Source: CAD feature listing. Evaluate the final solid. Frame: model axes, mm. Face numbers are marked on the shaded views. A direction names the side the tool comes from. Give positions to 0.01 mm unless a question says otherwise; leave off trailing zeros. Loops run counter-clockwise (first coordinate to the right, second up) from the corner with the lowest first, then second, coordinate; pieces in that order, holes last. Notation, with made-up numbers: M 82,39.5 L 88,39.5 A4 cw 88,45.5 Z; hole C 69,18.5 d6. An arc over 180 degrees is marked long. Answer in a Markdown table with one row per item.
```python
from build123d import *

# Parameters (mm, degrees)
F0_R      = 9.525
F1_DEPTH  = 1.905
F2_DEPTH  = 11.43
F6_R      = 0.635
F7_DEPTH  = 2.54
F10_W     = 10.16
F10_H     = 1.27
F11_DEPTH = 3.81
F12_W     = 10.16
F12_H     = 1.905
F13_DEPTH = 3.81
F15_DEPTH = 0.254
F17_DEPTH = 0.254


with BuildPart() as f1:
    # F0 (on Top) → F1 (new body)
    with BuildSketch(Plane.XY):
        Polygon((12.573, 7.2590249345), (0, 14.518049869), (-12.573, 7.2590249345), (-12.573, -7.2590249345), (0, -14.518049869), (12.573, -7.2590249345), align=None)
        Circle(F0_R, mode=Mode.SUBTRACT)
        Circle(F0_R)
        with BuildLine():
            ThreePointArc((-6.985, -3.4925), (-9.2723234913, 0), (-6.985, 3.4925))
            Line((-6.985, 3.4925), (-6.985, -3.4925))
        make_face(mode=Mode.SUBTRACT)
        with BuildLine():
            Line((6.985, -3.4925), (6.985, 3.4925))
            ThreePointArc((6.985, 3.4925), (9.2723234913, 0), (6.985, -3.4925))
        make_face(mode=Mode.SUBTRACT)
    extrude(amount=F1_DEPTH)

    # F0 (on Top) → F2 (join)
    with BuildSketch(Plane.XY):
        with BuildLine():
            Line((-6.985, -3.4925), (-6.985, 3.4925))
            ThreePointArc((-6.985, 3.4925), (-9.2723234913, 0), (-6.985, -3.4925))
        make_face()
        with BuildLine():
            ThreePointArc((6.985, -3.4925), (9.2723234913, 0), (6.985, 3.4925))
            Line((6.985, 3.4925), (6.985, -3.4925))
        make_face()
    extrude(amount=F2_DEPTH)

    # F4 (on offset) → F5 (revolve)
    with BuildSketch(Plane.XY.offset(9.525)):
        with BuildLine():
            ThreePointArc((0, 7.112), (-7.112, 0), (0, -7.112))
            Line((0, -7.112), (0, 7.112))
        make_face()
    revolve(axis=Axis((0, 0, 9.525), (0, 1, 0)))

    # F6
    f6_edges = [f1.edges().sort_by_distance(p)[0] for p in [
        (-6.985, 0, 11.43),
        (-9.272323, 0, 11.43),
        (6.985, 0, 11.43),
        (9.272323, 0, 11.43),
    ]]
    fillet(f6_edges, radius=F6_R)

    # F0 (on Top) → F7 (join)
    with BuildSketch(Plane.XY):
        Circle(F0_R)
        with BuildLine():
            ThreePointArc((-6.985, -3.4925), (-9.2723234913, 0), (-6.985, 3.4925))
            Line((-6.985, 3.4925), (-6.985, -3.4925))
        make_face(mode=Mode.SUBTRACT)
        with BuildLine():
            Line((6.985, -3.4925), (6.985, 3.4925))
            ThreePointArc((6.985, 3.4925), (9.2723234913, 0), (6.985, -3.4925))
        make_face(mode=Mode.SUBTRACT)
    extrude(amount=F7_DEPTH)

    # F10 (on line) → F11 (cut, symmetric)
    with BuildSketch(Plane(origin=(0, -2.38125, 8.8869459855), x_dir=(1, 0, 0), z_dir=(0, -0.2588190451, 0.9659258263))):
        with Locations((0, -4.318)):
            Rectangle(F10_W, F10_H)
    extrude(amount=F11_DEPTH, both=True, mode=Mode.SUBTRACT)

    # F12 (on line) → F13 (cut, symmetric)
    with BuildSketch(Plane(origin=(0, 2.38125, 8.8869459855), x_dir=(1, 0, 0), z_dir=(0, -0.2588190451, -0.9659258263))):
        with Locations((0, 9.4615)):
            Rectangle(F12_W, F12_H)
    extrude(amount=F13_DEPTH, both=True, mode=Mode.SUBTRACT)

    # F14 (on face) → F15 (cut)
    with BuildSketch(Plane(origin=(0, -3.5575048182, -0.9532305431), x_dir=(1, 0, 0), z_dir=(0, -0.9659258263, -0.2588190451))):
        with BuildLine():
            Line((3.0137271476, 10.2578568757), (-3.0137271476, 10.2578568757))
            ThreePointArc((-3.0137271476, 10.2578568757), (0, 6.0065940348), (3.0137271476, 10.2578568757))
        make_face()
    extrude(amount=-F15_DEPTH, mode=Mode.SUBTRACT)

    # F16 (on face) → F17 (cut)
    with BuildSketch(Plane(origin=(0, -8.2190628559, 2.2022912548), x_dir=(1, 0, 0), z_dir=(0, -0.9659258263, 0.2588190451))):
        Polygon((-3.2726924104, 9.7850203216), (-2.8154924104, 7.7530203216), (2.8154924104, 7.7530203216), (3.2726924104, 9.7850203216), (1.482303227, 12.3142628983), (-1.482303227, 12.3142628983), align=None)
    extrude(amount=-F17_DEPTH, mode=Mode.SUBTRACT)


solid = f1.part
```
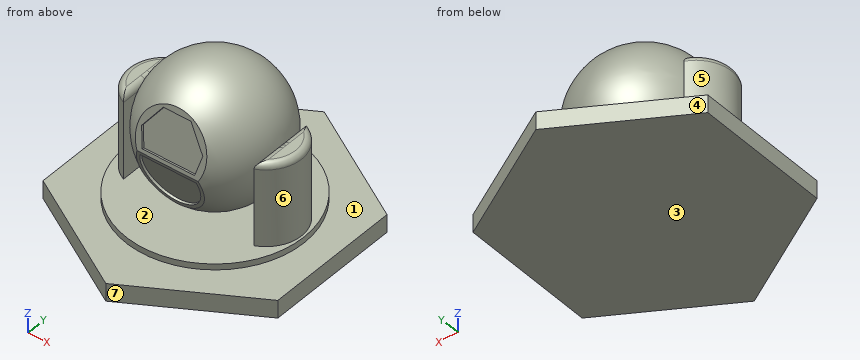
Q1. Section query C-C (y = -8.75). Output: boundary loops of the cut face in (x, z) (3 decimals), plus the area to 3 significant figures.
Values follow:
| item | result |
|---|---|
| outline | M -9.991,0 L 9.991,0 L 9.991,1.905 L 3.763,1.905 L 3.763,2.54 L -3.763,2.54 L -3.763,1.905 L -9.991,1.905 Z |
| area | 42.8 mm^2 |
Q2. Section query B-B (y = -4.25). Output: boundary loops of the cut face in (x, z) (3 decimals), plus the area to 3 significant figures.
Values follow:
| item | result |
|---|---|
| outline | M -12.573,0 L 12.573,0 L 12.573,1.905 L 8.524,1.905 L 8.524,2.54 L -8.524,2.54 L -8.524,1.905 L -12.573,1.905 Z; C 0,9.525 d11.405 |
| area | 161 mm^2 |
Q3. Reachability of the marked faces 5, 6 and 7 from +Z, -Z, +X, -X, +Y, -Y: full face, straight path, thin tool, end or side. Return the list, or none.
Values follow:
| item | result |
|---|---|
| face 5 | +Z, -X |
| face 6 | +Z, +X |
| face 7 | +Z, -Z, +X, -Y |
Q4. Contact query for flat-ended pins moving along their axis: pin 1 Ø1 at (x, y) = (6.5, 0) entering from +Z; pin 2 Ø2 at (x, z) = (3, 6.5) entering from +Y; pin 3 Ø5.5 at (x, y) = (-2, -2.5) entering from +Z. Output: stop coordinate, or through.
Values follow:
| item | result |
|---|---|
| pin 1 | z = 13.34 |
| pin 2 | y = 6.32 |
| pin 3 | z = 16.62 |
Q5. Mould query, pull axis Z, two halves, no side actions, for the marked faces 1, 2, 3 and 4. Classes: +Z half, -Z half, draft (parallel to the pull), parting line (faces both ways), or undercut.
Values follow:
| item | result |
|---|---|
| face 1 | +Z half |
| face 2 | undercut |
| face 3 | -Z half |
| face 4 | draft |
Q6. Ray query, probe 1 along X at (y, z) = (-2.25, 5.75) (3 decimals); probe 2 along Z at (x, y) = (11, -3) (3 decimals); probe 3 along Z at (x, y) = (5.75, 5.5). Return the intervals inside material, ascending. Write a range as from..to.
Values follow:
| item | result |
|---|---|
| probe 1 | -8.537..-6.985, -5.592..5.592, 6.985..8.537 |
| probe 2 | 0..1.905 |
| probe 3 | 0..2.54 |
Q7. Section query D-D (z = 8). Give the number of separate pieces and of enclosed holes in the cut face, plus the area to 3 significant figures.
Values follow:
| item | result |
|---|---|
| separate pieces | 3 |
| enclosed holes | 0 |
| area | 168 mm^2 |
Q8. Section query A-A (x = 6.25). Output: boundary loops of the cut face in (y, z) (3 decimals).
Values follow:
| item | result |
|---|---|
| outline | M -10.91,0 L 10.91,0 L 10.91,1.905 L 7.188,1.905 L 7.188,2.54 L -7.188,2.54 L -7.188,1.905 L -10.91,1.905 Z; C 0,9.525 d6.788 |
